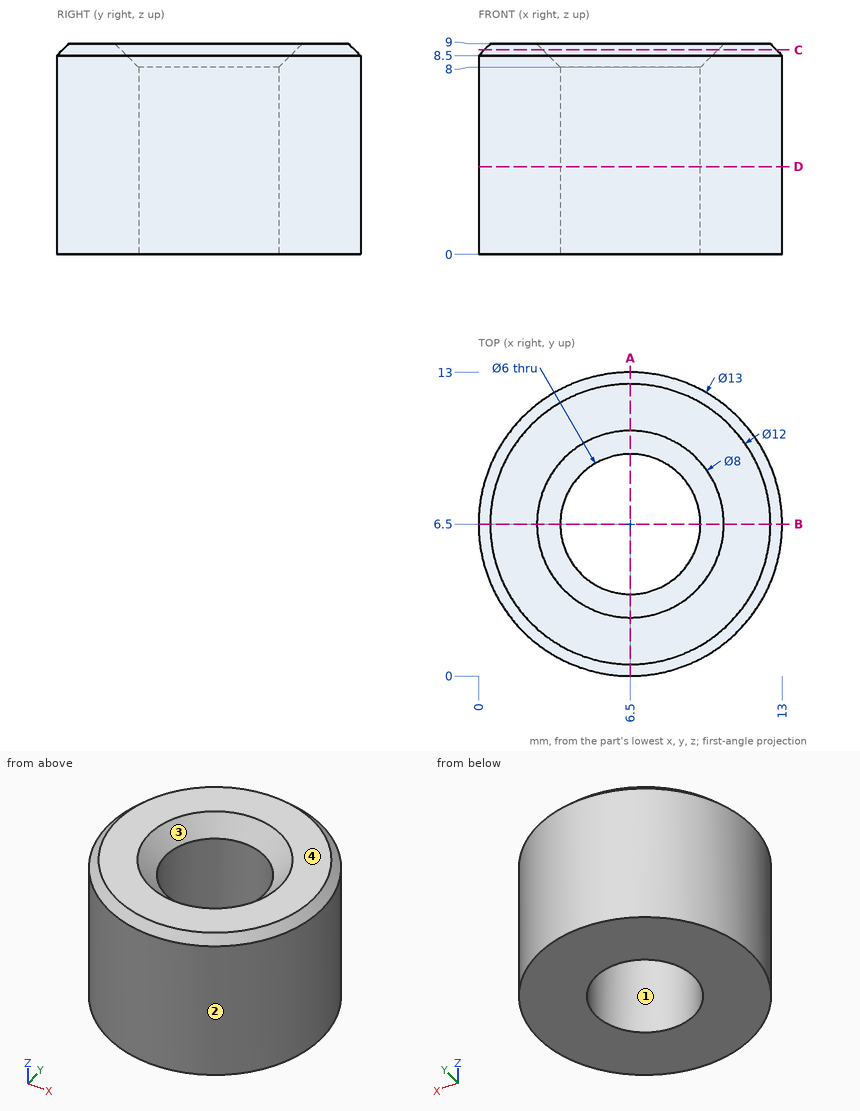
Source: three-view drawing plus pictorial views. Frame: mm from the lowest corner of the part. Coordinates: 2 decimals unless noted, no trailing zeros. Loops run counter-clockwise (first coordinate to the right, second up) from the corner with the lowest first, then second, coordinate; pieces in that order, holes last. Notation, with made-up numbers: (24.5, 43) - (71.5, 43) arc R14 cw to (71.5, 47) - close; hole circle Ø9 at (-15, 7). An arc over 180 degrees is marked (long way). One line per item, written item: value. Start each with the question number.
1. Contact query for flat-ended pins moving along their axis: P1, Ø1.5, axis at x = 11, z = 5.5, coming from the +Y side; P2, Ø5, axis at y = 2.5, z = 6, coming from the -X side; P3, Ø2, axis at x = 8, z = 3, coming from the +Y side. Output: stop coordinate, or through.
2. Ray query, L1, parallel to Y at x = 6.5, z = 5.25; L2, parallel to X at y = 8, z = 8.25; L3, parallel to X at y = 5.25, z = 4. Return the intervals inside material, ascending.
3. Mould query, pull axis Y, two halves, no side actions, for the marked faces 1, 2, 3 and 4. Classes: pulls with the +Y half, pulls with the -Y half, needs draft (parallel to the pull), parting line crosses it, or undercut.
4. Section C-C (z = 8.75). Return the cut outline in (x, y).
5. Section D-D (z = 3.75). Return the cut outline in (x, y).
6. Section A-A (x = 6.5). Return the cut outline in (y, z).
Verdict:
1. P1: stops at y = 11.81
1. P2: stops at x = 0.18
1. P3: stops at y = 12.98
2. L1: y = 0 to 3.5, 9.5 to 13
2. L2: x = 0.18 to 3.62, 9.38 to 12.82
2. L3: x = 0.12 to 3.77, 9.23 to 12.88
3. face 1: undercut
3. face 2: parting line crosses it
3. face 3: undercut
3. face 4: needs draft
4. outline: circle Ø12.5 at (6.5, 6.5); hole circle Ø7.5 at (6.5, 6.5)
5. outline: circle Ø13 at (6.5, 6.5); hole circle Ø6 at (6.5, 6.5)
6. outline: (0, 0) - (3.5, 0) - (3.5, 8) - (2.5, 9) - (0.5, 9) - (0, 8.5) - close; (9.5, 0) - (13, 0) - (13, 8.5) - (12.5, 9) - (10.5, 9) - (9.5, 8) - close
